from build123d import *

# Parameters (mm, degrees)
F0_R      = 6
F1_DEPTH  = 3
F2_R      = 4.8
F3_DEPTH  = 1.15
F4_R      = 6
F4_R_2    = 4.8
F5_DEPTH  = 20
F6_R      = 8
F6_R_2    = 6
F7_DEPTH  = 890
F8_R      = 6
F9_DEPTH  = 20
F10_R     = 4.8
F11_DEPTH = 1.15
F12_R     = 6
F12_R_2   = 4.8
F13_DEPTH = 3
F14_R     = 5
F15_DEPTH = 15
F16_SIZE  = 1


with BuildPart() as f1:
    # F0 (on Top) → F1 (new body)
    with BuildSketch(Plane.XY):
        Circle(F0_R)
    extrude(amount=F1_DEPTH)

    # F2 (on face) → F3 (join)
    with BuildSketch(Plane.XY.offset(3)):
        Circle(F2_R)
    extrude(amount=F3_DEPTH)

    # F4 (on face) → F5 (join)
    with BuildSketch(Plane.XY.offset(4.15)):
        Circle(F4_R)
        Circle(F4_R_2, mode=Mode.SUBTRACT)
        Circle(F4_R_2)
    extrude(amount=F5_DEPTH)

    # F6 (on face) → F7 (join)
    with BuildSketch(Plane.XY.offset(24.15)):
        Circle(F6_R)
        Circle(F6_R_2, mode=Mode.SUBTRACT)
        Circle(F6_R_2)
    extrude(amount=F7_DEPTH)

    # F8 (on face) → F9 (join)
    with BuildSketch(Plane.XY.offset(914.15)):
        Circle(F8_R)
    extrude(amount=F9_DEPTH)

    # F10 (on face) → F11 (join)
    with BuildSketch(Plane.XY.offset(934.15)):
        Circle(F10_R)
    extrude(amount=F11_DEPTH)

    # F12 (on face) → F13 (join)
    with BuildSketch(Plane.XY.offset(935.3)):
        Circle(F12_R)
        Circle(F12_R_2, mode=Mode.SUBTRACT)
        Circle(F12_R_2)
    extrude(amount=F13_DEPTH)

    # F14 (on face) → F15 (join)
    with BuildSketch(Plane.XY.offset(938.3)):
        Circle(F14_R)
    extrude(amount=F15_DEPTH)

    # F16
    f16_edges = [f1.edges().sort_by_distance(p)[0] for p in [
        (-5, 0, 953.3),
        (-6, 0, 0),
    ]]
    chamfer(f16_edges, length=F16_SIZE)


solid = f1.part
Could you check a few things on this model? Use its own coordinates, in mm. A direction names the side the tool comes from. Give positions to 0.01 mm unless a question says otherwise; leave off trailing zeros. Order: outer loops, then holes, each group sorted by start corner. A loop starts at its lowest first (then second) coordinate and runs counter-clockwise, first axis right, second up. Notation, with made-up numbers: (85.5, 5) -> (99.5, 5) arc R32 ccw to (99.5, 36) -> close; hole circle Ø1 at (73.25, 35.25). An arc over 180 degrees is marked (long way). Return JSON: item names as keys, results as strings.
1. I need wall thicknesses on line 1 (Z direction, x = -3.5, y = 3.5); line 2 (Z direction, x = 3, y = -4.5); line 3 (Y direction, x = 1.5, z = 814). Which ranges of each line are inside material? Lowest first, please. Write a range as from..to.
Answer list:
{"line 1": "z = 0..3, 4.15..934.15, 935.3..952.35", "line 2": "z = 0.41..3, 4.15..934.15, 935.3..938.3", "line 3": "y = -7.86..7.86"}
2. Imagine slicing it at A-A on z = 562. List the corners of the cut face in (x, y) for me.
Answer list:
{"outline": "circle Ø16 at (0, 0)"}
3. For pin 1 Ø2 at (x, y) = (5.5, 4.5) entering from -Z; pin 2 Ø6 at (y, z) = (6, 656) entering from +X; pin 3 Ø3 at (x, z) = (5, 306) entering from -Y, each with a flat end and sliding along its axis, tell me the tip position at first contact or that it passes through.
Answer list:
{"pin 1": "stops at z = 24.15", "pin 2": "stops at x = 7.42", "pin 3": "stops at y = -7.19"}
4. On a 3-axis mill with a long thin cutter (end or side, diameter ignored), from which of +Z, -Z, +X, -X, +Y, -Y can I reach the whole of each face in a straight line? I mean faces 1 (the cylindrical face through (-1.73, -7.81, 462.92)), 2 (the flat face through (-2, 6, 24.15)), 3 (the flat face through (-2, 6, 914.15)). Say none if no direction works.
Answer list:
{"face 1": "+Z, -Z", "face 2": "-Z", "face 3": "+Z"}
